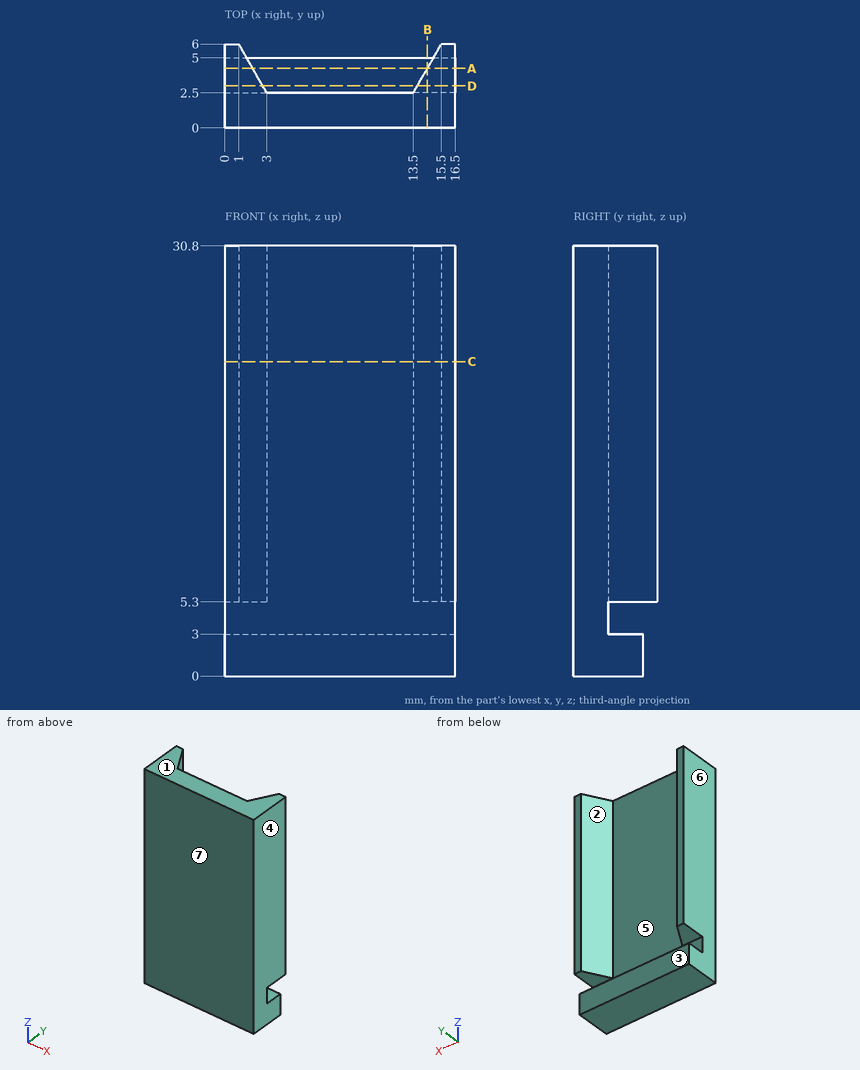
Input: dimensioned drawing with shaded views. Units: mm. Origin: part minimum x, y, z. A direction names the side the tool comes from. Give positions to 0.01 mm unless a question says otherwise; leave off trailing zeros. Loops run counter-clockwise (first coordinate to the right, second up) from the corner with the lowest first, then second, coordinate; pieces in that order, holes last. Notation, with made-up numbers: (31.5, 32) -> (69.5, 32) arc R21 cw to (69.5, 67) -> close; hole circle Ø9 at (21.5, 11). An arc over 180 degrees is marked (long way). Return JSON: item names as keys, results as strings.
Item 1: Access query for the marked faces 1, 2 and 3. Directions: +Z, -Z, +X, -X, +Y, -Y. A direction counts if a zero-diameter tool reaches every point of the face in a straight line with its end or side. Return the directions, or none.
Filled in:
{"face 1": "+Z, +X, -X, +Y, -Y", "face 2": "+Z, +Y", "face 3": "-Z, +X, -X, +Y"}
Item 2: Section C-C, the plane z = 22.5. Output: boundary loops of the cut face in (x, y).
Filled in:
{"outline": "(0, 0) -> (16.5, 0) -> (16.5, 6) -> (15.5, 6) -> (13.5, 2.5) -> (3, 2.5) -> (1, 6) -> (0, 6) -> close"}
Item 3: Section A-A, the plane y = 4.25. Output: boundary loops of the cut face in (x, z), plus the area to 4 significant figures.
Filled in:
{"outline": "(0, 0) -> (16.5, 0) -> (16.5, 3) -> (0, 3) -> close; (0, 5.3) -> (2, 5.3) -> (2, 30.8) -> (0, 30.8) -> close; (14.5, 5.3) -> (16.5, 5.3) -> (16.5, 30.8) -> (14.5, 30.8) -> close", "area": "151.5 mm^2"}
Item 4: Mould query, pull axis X, two halves, no side actions, for the marked faces 4, 5, 6 and 7. Classes: released by +X, released by -X, zero draft, split by the parting line, or undercut.
Filled in:
{"face 4": "released by +X", "face 5": "undercut", "face 6": "released by -X", "face 7": "zero draft"}
Item 5: Pin query (flat end, axial travel): P1, Ø1, axis at x = 5, z = 24, coming from the -Y side; P2, Ø0.9, axis at x = 6, z = 2, coming from the +Y side. Return the tip coordinate at first contact, or that it passes through.
Filled in:
{"P1": "y = 0", "P2": "y = 5"}
Item 6: Section B-B, the plane x = 14.5. Output: boundary loops of the cut face in (y, z), plus the area to 3 significant figures.
Filled in:
{"outline": "(0, 0) -> (5, 0) -> (5, 3) -> (2.5, 3) -> (2.5, 5.3) -> (4.25, 5.3) -> (4.25, 30.8) -> (0, 30.8) -> close", "area": "129 mm^2"}
Item 7: Line query: line 1 (Z direction, x = 14.75, y = 4); line 2 (Z direction, x = 2.25, y = 4.5); line 3 (X direction, y = 3.5, z = 20). Output: solid intervals per line, ascending.
Filled in:
{"line 1": "0 to 3, 5.3 to 30.8", "line 2": "0 to 3", "line 3": "0 to 2.43, 14.07 to 16.5"}
Item 8: Section D-D, the plane y = 3. Output: boundary loops of the cut face in (x, z), plus the area to 3 significant figures.
Filled in:
{"outline": "(0, 0) -> (16.5, 0) -> (16.5, 3) -> (0, 3) -> close; (0, 5.3) -> (2.71, 5.3) -> (2.71, 30.8) -> (0, 30.8) -> close; (13.79, 5.3) -> (16.5, 5.3) -> (16.5, 30.8) -> (13.79, 30.8) -> close", "area": "188 mm^2"}
